from build123d import *

# Parameters (mm, degrees)
F0_R     = 28.575
F1_DEPTH = 19.05
F2_R     = 6.35
F3_DEPTH = 19.051


with BuildPart() as f1:
    # F0 (on Top) → F1 (new body)
    with BuildSketch(Plane.XY):
        with BuildLine():
            ThreePointArc((-50.8, -165.1), (-45.220384, -178.570384), (-31.75, -184.15))
            Line((-31.75, -184.15), (31.75, -184.15))
            ThreePointArc((31.75, -184.15), (45.220384, -178.570384), (50.8, -165.1))
            Line((50.8, -165.1), (50.8, 77.47))
            ThreePointArc((50.8, 77.47), (47.080256, 86.450256), (38.1, 90.17))
            Line((38.1, 90.17), (34.925337, 90.17))
            ThreePointArc((34.925337, 90.17), (24.14903, 94.633693), (19.685337, 105.41))
            Line((19.685337, 105.41), (19.685337, 168.91))
            ThreePointArc((19.685337, 168.91), (15.221645, 179.686307), (4.445337, 184.15))
            Line((4.445337, 184.15), (-4.445337, 184.15))
            ThreePointArc((-4.445337, 184.15), (-15.221645, 179.686307), (-19.685337, 168.91))
            Line((-19.685337, 168.91), (-19.685337, 105.41))
            ThreePointArc((-19.685337, 105.41), (-24.14903, 94.633693), (-34.925337, 90.17))
            Line((-34.925337, 90.17), (-38.1, 90.17))
            ThreePointArc((-38.1, 90.17), (-47.080256, 86.450256), (-50.8, 77.47))
            Line((-50.8, 77.47), (-50.8, -165.1))
        make_face()
        with Locations((0, -146.05)):
            Circle(F0_R, mode=Mode.SUBTRACT)
        with Locations((0, -78.74)):
            Circle(F0_R, mode=Mode.SUBTRACT)
        with Locations((0, -11.43)):
            Circle(F0_R, mode=Mode.SUBTRACT)
        with Locations((0, 55.88)):
            Circle(F0_R, mode=Mode.SUBTRACT)
    extrude(amount=F1_DEPTH)

    # F2 (on face) → F3 (cut, through all)
    with BuildSketch(Plane.XY.offset(19.05)):
        with Locations((0, 168.91)):
            Circle(F2_R)
    extrude(amount=-F3_DEPTH, mode=Mode.SUBTRACT)


solid = f1.part
Source: CAD feature listing. Evaluate the final solid. Frame: model axes, mm. A direction names the side the tool comes from. Round coordinates to 2 decimals unless told otherwise and drop trailing zeros. Order: outer loops, then holes, each group sorted by start corner. A loop starts at its lowest first (then second) coordinate and runs counter-clockwise, first axis right, second up. Notation, with made-up numbers: (8.25, 79.5) -> (26.25, 79.5) arc R25 ccw to (26.25, 108.5) -> close; hole circle Ø7 at (-14, 13.5). An arc over 180 degrees is marked (long way). Answer as CSV lines item,"result".
Item 1: Pin query (flat end, axial travel): pin 1 Ø1 at (x, z) = (-36, 11.5) entering from +Y; pin 2 Ø20.5 at (x, y) = (0, 168.91) entering from -Z; pin 3 Ø3 at (y, z) = (105, 15.5) entering from +X; pin 4 Ø4 at (x, z) = (34, 3) entering from +Y. Return the tip coordinate at first contact, or that it passes through.
A:
pin 1,"y = 90.17"
pin 2,"z = 0"
pin 3,"x = 19.81"
pin 4,"y = 90.45"
Item 2: Section B-B, the plane y = 55.88. Return loops of the section in (x, z) (3 decimals).
A:
outline,"(-50.8, 0) -> (-28.575, 0) -> (-28.575, 19.05) -> (-50.8, 19.05) -> close; (28.575, 0) -> (50.8, 0) -> (50.8, 19.05) -> (28.575, 19.05) -> close"
Item 3: Section D-D, the plane y = -131. Return loops of the section in (x, z).
A:
outline,"(-50.8, 0) -> (-24.29, 0) -> (-24.29, 19.05) -> (-50.8, 19.05) -> close; (24.29, 0) -> (50.8, 0) -> (50.8, 19.05) -> (24.29, 19.05) -> close"
Item 4: Line query: L1, parallel to Y at x = 0, z = 7.5 (3 decimals); L2, parallel to X at y = 168, z = 4.25; L3, parallel to Y at x = 25, z = 9. Output: solid intervals per line, ascending.
A:
L1,"-184.15 to -174.625, -117.475 to -107.315, -50.165 to -40.005, 17.145 to 27.305, 84.455 to 162.56, 175.26 to 184.15"
L2,"-19.69 to -6.28, 6.28 to 19.69"
L3,"-184.15 to -159.89, -132.21 to -92.58, -64.9 to -25.27, 2.41 to 42.04, 69.72 to 93.85"
Item 5: Reachability of faces 4 (the face through (-3.72, -50.41, 9.39)), 5 (the face through (-19.685, 138, 9)) from +Z, -Z, +X, -X, +Y, -Y: full face, straight path, thin tool, end or side. Return the list, or none.
A:
face 4,"+Z, -Z"
face 5,"+Z, -Z, -X, +Y"
Item 6: Pull-direction query (X, two-part tool) for faces 1 (the face through (-6.194, -39.325, 9.392)), 2 (the face through (19.685, 137, 9)), 3 (the face through (-24.031, 94.753, 9.392)); classes: pulls with the +X half, pulls with the -X half, needs draft (parallel to the pull), parting line crosses it, or undercut.
A:
face 1,"undercut"
face 2,"pulls with the +X half"
face 3,"pulls with the -X half"
Item 7: Section A-A, the plane x = 0. Return loops of the section in (y, z) (3 decimals), plus the area to 3 significant figures.
A:
outline,"(-184.15, 0) -> (-174.625, 0) -> (-174.625, 19.05) -> (-184.15, 19.05) -> close; (-117.475, 0) -> (-107.315, 0) -> (-107.315, 19.05) -> (-117.475, 19.05) -> close; (-50.165, 0) -> (-40.005, 0) -> (-40.005, 19.05) -> (-50.165, 19.05) -> close; (17.145, 0) -> (27.305, 0) -> (27.305, 19.05) -> (17.145, 19.05) -> close; (84.455, 0) -> (162.56, 0) -> (162.56, 19.05) -> (84.455, 19.05) -> close; (175.26, 0) -> (184.15, 0) -> (184.15, 19.05) -> (175.26, 19.05) -> close"
area,"2,420 mm²"
Item 8: Section C-C, the plane z = 7.5. Return loops of the section in (x, y) (3 decimals), plus the area to 3 significant figures.
A:
outline,"(-50.8, -165.1) arc R19.05 ccw to (-31.75, -184.15) -> (31.75, -184.15) arc R19.05 ccw to (50.8, -165.1) -> (50.8, 77.47) arc R12.7 ccw to (38.1, 90.17) -> (34.925, 90.17) arc R15.24 cw to (19.685, 105.41) -> (19.685, 168.91) arc R15.24 ccw to (4.445, 184.15) -> (-4.445, 184.15) arc R15.24 ccw to (-19.685, 168.91) -> (-19.685, 105.41) arc R15.24 cw to (-34.925, 90.17) -> (-38.1, 90.17) arc R12.7 ccw to (-50.8, 77.47) -> close; hole circle Ø57.15 at (0, -146.05); hole circle Ø57.15 at (0, -78.74); hole circle Ø57.15 at (0, -11.43); hole circle Ø57.15 at (0, 55.88); hole circle Ø12.7 at (0, 168.91)"
area,"21,000 mm²"
